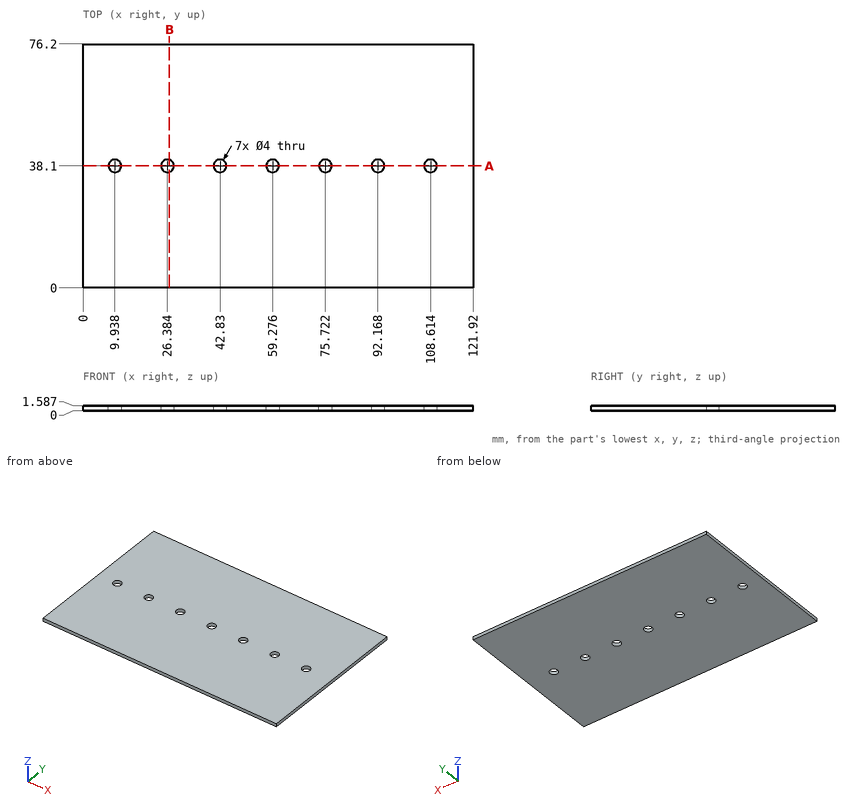
Design review of the part shown in the three views and the two pictorial views. Dimensions are in mm from the part's minimum x, y and z. Round coordinates to 2 decimals unless told otherwise and drop trailing zeros. Write each loop counter-clockwise with the first axis right and the second up, starting at its lowest first coordinate (ties: lowest second). Pieces come first, ordered by that corner, then holes.
1) For line 1 along Y through (x, z) = (43, 0.8); line 2 along Y through (x, z) = (75, 1.55) (1 decimal), list the stretches that pass through material, from the lowest coordinate up.
Answer below:
line 1: y = 0 to 36.11, 40.09 to 76.2
line 2: y = 0 to 36.2, 40 to 76.2
2) Take a section at A-A on y = 38.1. State how many separate pieces and enclosed holes the cut face has, then the cut area to 3 significant figures.
Answer below:
separate pieces: 8
enclosed holes: 0
area: 149 mm2
3) Insertion check: pin 1 Ø2.5 at (x, y) = (75.72, 38.1) entering from -Z. The pin has a flat end and moves straight along its axis. Give the tip position at first contact, or say it passes through.
Answer below:
pin 1: passes through
4) Take a section at B-B on x = 27. Give the boundary of the cut face in (y, z).
Answer below:
outline: (0, 0) - (36.2, 0) - (36.2, 1.59) - (0, 1.59) - close; (40, 0) - (76.2, 0) - (76.2, 1.59) - (40, 1.59) - close
